Model file for the job. Use its own axes, mm. Face numbers are marked on the shaded views. A direction names the side the tool comes from. Give positions to 0.01 mm unless a question says otherwise; leave off trailing zeros. Order: outer loops, then holes, each group sorted by start corner. A loop starts at its lowest first (then second) coordinate and runs counter-clockwise, first axis right, second up. Notation, with made-up numbers: (-3, 41.25) - (27, 41.25) arc R21 cw to (27, 68.25) - close; hole circle Ø10 at (-38, -1). An arc over 180 degrees is marked (long way). Use CSV: the item, a comma, the result in double quotes. Start each with the question number.
(1) Band-saw the part on A-A, the plane x = 0. Give the cut face in (y, z), then the cut area to 3 significant figures.
(2) Probe L1, parallel to Z at x = 0, y = -3.75; L2, parallel to Y at x = 10.5, z = 1; L3, parallel to Z at x = 0, y = -0.8. List the from-to ranges inside material, lowest first.
(3) Band-saw the part on D-D, the plane x = 7.5. Give the cut face in (y, z), then the cut area to 3 significant figures.
(4) Tool access for the marked faces 1, 2, 3 and 4: list every direction of +Z, -Z, +X, -X, +Y, -Y with a clear straight run to the whole face (end or side of a thin tool).
(5) Band-saw the part on B-B, the plane y = -6.5. Give the cut face in (x, z).
(6) Pull direction X, two halves, no side cores. Call the marked faces 5, 6 and 7: +X half, -X half, draft (parallel to the pull), parting line (faces both ways), or undercut.
(7) Band-saw the part on C-C, the plane y = -10. Give the cut face in (x, z), then the cut area to 3 significant figures.
(8) Drop flat-ended pins along their axis: pin 1 Ø1 at (x, z) = (-6.5, -0.5) entering from -Y; pin 2 Ø5 at (x, y) = (2.5, -3.5) entering from +Z; pin 3 Ø1.9 at (x, y) = (0.5, -7) entering from -Z. Give the stop position or say it passes through.
from build123d import *

# Parameters (mm, degrees)
F0_R      = 11.5
F0_R_2    = 3
F0_R_3    = 1.8
F1_DEPTH  = 1.5
F2_R      = 1.65
F2_R_2    = 3
F3_DEPTH  = 6.5
F3_FACE_R = 3
F4_DEPTH  = 4
F5_R      = 1.25
F6_DEPTH  = 2


with BuildPart() as f1:
    # F0 (on Front) → F1 (new body)
    with BuildSketch(Plane.XZ):
        Circle(F0_R)
        Circle(F0_R_2, mode=Mode.SUBTRACT)
        with Locations((6.5, 0)):
            Circle(F0_R_3, mode=Mode.SUBTRACT)
        Circle(F0_R_2)
        with Locations((6.5, 0)):
            Circle(F0_R_3)
    extrude(amount=F1_DEPTH)

    # F2 (on face) → F3 (join)
    with BuildSketch(Plane.XZ.offset(1.5)):
        with Locations((-6.8, 0)):
            Circle(F2_R)
        Circle(F2_R_2)
        with BuildLine():
            ThreePointArc((1.873499, 0.7), (1.968121, 0.355669), (2, 0))
            ThreePointArc((2, 0), (-0.355669, -1.968121), (-1.873499, 0.7))
            ThreePointArc((-1.873499, 0.7), (0, 2), (1.873499, 0.7))
        make_face(mode=Mode.SUBTRACT)
        with BuildLine():
            Line((-1.873499, 0.7), (1.873499, 0.7))
            ThreePointArc((1.873499, 0.7), (0, 2), (-1.873499, 0.7))
        make_face()
        with Locations((6.8, 0)):
            Circle(F2_R)
    extrude(amount=F3_DEPTH)

    # F3_face (on face) → F4 (join)
    with BuildSketch(Plane(origin=(0, -8, 0.227747), x_dir=(1, 0, 0), z_dir=(0, -1, 0))):
        with Locations((0, -0.227747)):
            Circle(F3_FACE_R)
        with BuildLine():
            ThreePointArc((1.873499, 0.472253), (0, -2.227747), (-1.873499, 0.472253))
            Line((-1.873499, 0.472253), (1.873499, 0.472253))
        make_face(mode=Mode.SUBTRACT)
    extrude(amount=F4_DEPTH)

    # F5 (on face) → F6 (cut)
    with BuildSketch(Plane(origin=(0, 0, 0), x_dir=(-1, 0, 0), z_dir=(0, 1, 0))):
        Circle(F5_R)
    extrude(amount=-F6_DEPTH, mode=Mode.SUBTRACT)


solid = f1.part
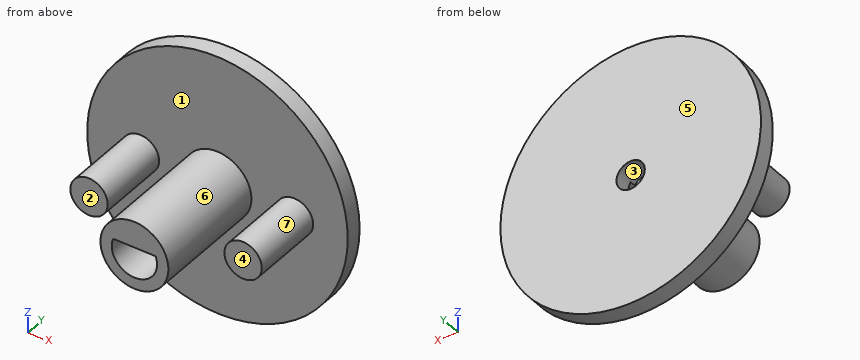
Answer block:
1,outline,"(-12, -3) - (-1.5, -3) - (-1.5, -11.5) - (0, -11.5) - (0, -1.25) - (-1.5, -1.25) - (-1.5, -2) - (-12, -2) - close; (-12, 0.7) - (-2, 0.7) - (-2, 1.25) - (0, 1.25) - (0, 11.5) - (-1.5, 11.5) - (-1.5, 3) - (-12, 3) - close"
1,area,"65.1 mm2"
2,L1,"z = -3 to -2, 0.7 to 3"
2,L2,"y = -1.5 to 0"
2,L3,"z = -11.5 to -1.25, 1.25 to 11.5"
3,outline,"(-8, -1.49) - (-1.5, -1.49) - (-1.5, -8.72) - (0, -8.72) - (0, 8.72) - (-1.5, 8.72) - (-1.5, 1.49) - (-8, 1.49) - close"
3,area,"45.6 mm2"
4,face 1,"-Y"
4,face 2,"+Z, -Z, -X, -Y"
4,face 3,"+Y"
4,face 4,"+Z, -Z, +X, -Y"
5,outline,"circle Ø3.3 at (-6.8, 0); circle Ø6 at (0, 0); circle Ø3.3 at (6.8, 0); hole (-1.87, 0.7) arc R2 ccw (long way) to (2, 0) arc R2 ccw to (1.87, 0.7) - close"
6,face 5,"draft"
6,face 6,"undercut"
6,face 7,"undercut"
7,outline,"circle Ø6 at (0, 0); hole (-1.87, 0.7) arc R2 ccw (long way) to (1.87, 0.7) - close"
7,area,"19.2 mm2"
8,pin 1,"stops at y = -8"
8,pin 2,"stops at z = 11.46"
8,pin 3,"stops at z = -3"
